```python
from build123d import *

# Parameters (mm, degrees)
F1_DEPTH = 20
F2_R     = 10
F3_DEPTH = 36
F4_R     = 22.5
F4_R_2   = 10
F5_DEPTH = 4
F7_D     = 3.3
F7_DEPTH = 10
F7_TIP   = 0.9914200214
F9_D     = 2.7
F9_DEPTH = 15
F9_TIP   = 0.8111618357


with BuildPart() as f1:
    # F0 (on Top) → F1 (new body)
    with BuildSketch(Plane.XY):
        with BuildLine():
            ThreePointArc((-22.5, 0), (0, -22.5), (22.5, 0))
            ThreePointArc((22.5, 0), (0, 22.5), (-22.5, 0))
        make_face()
    extrude(amount=F1_DEPTH)

    # F2 (on face) → F3 (join)
    with BuildSketch(Plane.XY.offset(20)):
        Circle(F2_R)
    extrude(amount=F3_DEPTH)

    # F4 (on face) → F5 (join)
    with BuildSketch(Plane.XY.offset(56)):
        Circle(F4_R)
        Circle(F4_R_2, mode=Mode.SUBTRACT)
        Circle(F4_R_2)
    extrude(amount=F5_DEPTH)

    # F7
    with Locations(Plane.XY.offset(60)):
        with Locations((0, 17), (14.7224318643, -8.5), (-14.7224318643, -8.5)):
            Hole(F7_D / 2, depth=F7_DEPTH)
            with Locations((0, 0, -(F7_DEPTH + F7_TIP / 2))):  # 118° drill point
                Cone(0, F7_D / 2, F7_TIP, mode=Mode.SUBTRACT)

    # F9
    with Locations(Plane(origin=(0, 0, 0), x_dir=(1, 0, 0), z_dir=(0, 0, -1))):
        with Locations((14.7224318643, -8.5), (-14.7224318643, -8.5), (0, 17)):
            Hole(F9_D / 2, depth=F9_DEPTH)
            with Locations((0, 0, -(F9_DEPTH + F9_TIP / 2))):  # 118° drill point
                Cone(0, F9_D / 2, F9_TIP, mode=Mode.SUBTRACT)


solid = f1.part
```
Geometry check sheet. Reference: the model listing, model coordinates, mm. A direction names the side the tool comes from. Round coordinates to 2 decimals unless told otherwise and drop trailing zeros. Loops run counter-clockwise (first coordinate to the right, second up) from the corner with the lowest first, then second, coordinate; pieces in that order, holes last. Notation, with made-up numbers: (-13.75, 34.25) - (7.25, 34.25) arc R4 cw to (7.25, 40.25) - close; hole circle Ø8 at (-30, 3.5). An arc over 180 degrees is marked (long way). Write item = value, one per line. Start each with the question number.
1. Thickness scan on line 1 (Z direction, x = -12, y = 8.5); line 2 (Y direction, x = 0, z = 9); line 3 (Y direction, x = 0, z = 58.55). Record the ranges inside material, lowest first.
2. Section check A-A on x = 18. Enter the section's corners in (y, z).
3. Set-up check for faces 1 (the face through (-0.89, 18.39, 57.97)), 2 (the face through (0.176, -18.339, 7.605)), 3 (the face through (-2.17, -9.76, 37.75)): record each of +Z, -Z, +X, -X, +Y, -Y from which the full face is reachable in a straight line by a thin tool's end or side.
4. Section check B-B on y = 13.5. Enter the section's corners in (x, z), then the cut area to 3 significant figures.
5. Depth check by flat-ended pin: pin 1 (10 mm diameter, centred on x = -11, y = 15, fed in from -Z); pin 2 (2 mm diameter, centred on x = -4.5, z = 45.5, fed in from +Y); pin 3 (3 mm diameter, centred on x = -14.72, y = -8.5, fed in from +Z); pin 4 (8 mm diameter, centred on x = -8.5, z = 33.5, fed in from +Y). Enter the tip coordinate at first touch or a pass-through.
6. Mould release check, pull along Z, two halves, no side actions. Record for faces 4 (the face through (5, -10, 20)), 5 (the face through (13.15, -8, 57.97)), 6 (the face through (-0.17, -17.16, 15.67)): released by +Z, released by -Z, zero draft, split by the parting line, or undercut.
7. Section check D-D on z = 26.5. Enter the section's corners in (x, y), then the cut area to 3 significant figures.
8. Section check C-C on y = 0. Enter the section's corners in (x, z).
Working result:
q1.line_1 = 0 to 20, 56 to 60
q1.line_2 = -22.5 to -18.35, -15.65 to 22.5
q1.line_3 = -22.5 to 15.35, 18.65 to 22.5
q2.outline = (-13.5, 0) - (13.5, 0) - (13.5, 20) - (-13.5, 20) - close; (-13.5, 56) - (13.5, 56) - (13.5, 60) - (-13.5, 60) - close
q3.face_1 = +Z
q3.face_2 = -Z
q3.face_3 = none
q4.outline = (-18, 0) - (18, 0) - (18, 20) - (-18, 20) - close; (-18, 56) - (18, 56) - (18, 60) - (-18, 60) - close
q4.area = 864 mm^2
q5.pin_1 = 0
q5.pin_2 = 9.37
q5.pin_3 = 20
q5.pin_4 = 8.93
q6.face_4 = undercut
q6.face_5 = zero draft
q6.face_6 = released by -Z
q7.outline = circle Ø20 at (0, 0)
q7.area = 314 mm^2
q8.outline = (-22.5, 0) - (22.5, 0) - (22.5, 20) - (10, 20) - (10, 56) - (22.5, 56) - (22.5, 60) - (-22.5, 60) - (-22.5, 56) - (-10, 56) - (-10, 20) - (-22.5, 20) - close
